from build123d import *

# Parameters (mm, degrees)
SKETCH1_W            = 122
SKETCH1_H            = 101.3
BOSS_EXTRUDE1_DEPTH  = 18
SKETCH2_W            = 118
SKETCH2_H            = 97.3
CUT_EXTRUDE1_DEPTH   = 34
SKETCH4_R            = 5.953519792
CUT_EXTRUDE5_DEPTH   = 2
SKETCH5_W            = 41.658553798
SKETCH5_H            = 19.550778972
CUT_EXTRUDE10_DEPTH  = 2
SKETCH9_W            = 11.907039584
SKETCH9_H            = 11.615
CUT_EXTRUDE12_DEPTH  = 5
SKETCH10_W           = 11.907039584
SKETCH10_H           = 11.615
CUT_EXTRUDE13_DEPTH  = 5
SKETCH11_R           = 1.25
BOSS_EXTRUDE6_DEPTH  = 17
SKETCH14_R           = 1.25
BOSS_EXTRUDE8_DEPTH  = 17
SKETCH15_R           = 1.25
BOSS_EXTRUDE10_DEPTH = 17
SKETCH16_W           = 14.214546847
SKETCH16_H           = 17.568519792
CUT_EXTRUDE14_DEPTH  = 5
SKETCH17_R           = 1.6
BOSS_EXTRUDE11_DEPTH = 1
BOSS_EXTRUDE11_TAPER = 20
SKETCH18_R           = 1.6
BOSS_EXTRUDE13_DEPTH = 1
BOSS_EXTRUDE13_TAPER = 20
SKETCH19_R           = 1.513275
BOSS_EXTRUDE14_DEPTH = 1
BOSS_EXTRUDE14_TAPER = 20


with BuildPart() as part:
    # Sketch1 → Boss-Extrude1 (new, symmetric)
    with BuildSketch(Plane.XY):
        with Locations((129.5, -82.15)):
            Rectangle(SKETCH1_W, SKETCH1_H)
    extrude(amount=BOSS_EXTRUDE1_DEPTH, both=True)

    # Sketch2 → Cut-Extrude1 (cut)
    with BuildSketch(Plane.XY.offset(18)):
        with Locations((129.5, -82.15)):
            Rectangle(SKETCH2_W, SKETCH2_H)
    extrude(amount=-CUT_EXTRUDE1_DEPTH, mode=Mode.SUBTRACT)

    # Sketch4 → Cut-Extrude5 (cut)
    with BuildSketch(Plane(origin=(0, -132.8, 0), x_dir=(-1, 0, 0), z_dir=(0, -1, 0))):
        with Locations(Location((-132.2, -6.385, 0), (0, 0, 90))):
            Circle(SKETCH4_R)
        with Locations(Location((-146.414546847, -6.385, 0), (0, 0, 90))):
            Circle(SKETCH4_R)
    extrude(amount=-CUT_EXTRUDE5_DEPTH, mode=Mode.SUBTRACT)

    # Sketch5 → Cut-Extrude10 (cut)
    with BuildSketch(Plane(origin=(0, -132.8, 0), x_dir=(-1, 0, 0), z_dir=(0, -1, 0))):
        with Locations((-96.070620406, -8.224610514)):
            Rectangle(SKETCH5_W, SKETCH5_H)
    extrude(amount=-CUT_EXTRUDE10_DEPTH, mode=Mode.SUBTRACT)

    # Sketch9 → Cut-Extrude12 (cut)
    with BuildSketch(Plane(origin=(0, -132.8, 0), x_dir=(-1, 0, 0), z_dir=(0, -1, 0))):
        with Locations((-146.414546847, -12.1925)):
            Rectangle(SKETCH9_W, SKETCH9_H)
    extrude(amount=-CUT_EXTRUDE12_DEPTH, mode=Mode.SUBTRACT)

    # Sketch10 → Cut-Extrude13 (cut)
    with BuildSketch(Plane(origin=(0, -132.8, 0), x_dir=(-1, 0, 0), z_dir=(0, -1, 0))):
        with Locations((-132.2, -12.1925)):
            Rectangle(SKETCH10_W, SKETCH10_H)
    extrude(amount=-CUT_EXTRUDE13_DEPTH, mode=Mode.SUBTRACT)

    # Sketch11 → Boss-Extrude6 (add)
    with BuildSketch(Plane.XY.offset(-16)):
        with Locations((91.5, -40.5)):
            Circle(SKETCH11_R)
    extrude(amount=BOSS_EXTRUDE6_DEPTH)

    # Sketch14 → Boss-Extrude8 (add)
    with BuildSketch(Plane.XY.offset(-16)):
        with Locations((166.43, -40.5)):
            Circle(SKETCH14_R)
    extrude(amount=BOSS_EXTRUDE8_DEPTH)

    # Sketch15 → Boss-Extrude10 (add)
    with BuildSketch(Plane.XY.offset(-16)):
        with Locations((180.9, -126.3)):
            Circle(SKETCH15_R)
    extrude(amount=BOSS_EXTRUDE10_DEPTH)

    # Sketch16 → Cut-Extrude14 (cut)
    with BuildSketch(Plane(origin=(0, -132.8, 0), x_dir=(-1, 0, 0), z_dir=(0, -1, 0))):
        with Locations((-139.307273424, -9.215740104)):
            Rectangle(SKETCH16_W, SKETCH16_H)
    extrude(amount=-CUT_EXTRUDE14_DEPTH, mode=Mode.SUBTRACT)

    # Sketch17 → Boss-Extrude11 (add)
    with BuildSketch(Plane.XY.offset(-16)):
        with Locations((91.5, -40.5)):
            Circle(SKETCH17_R)
    extrude(amount=BOSS_EXTRUDE11_DEPTH, taper=BOSS_EXTRUDE11_TAPER)

    # Sketch18 → Boss-Extrude13 (add)
    with BuildSketch(Plane.XY.offset(-16)):
        with Locations((166.43, -40.5)):
            Circle(SKETCH18_R)
    extrude(amount=BOSS_EXTRUDE13_DEPTH, taper=BOSS_EXTRUDE13_TAPER)

    # Sketch19 → Boss-Extrude14 (add)
    with BuildSketch(Plane.XY.offset(-16)):
        with Locations((180.9, -126.3)):
            Circle(SKETCH19_R)
    extrude(amount=BOSS_EXTRUDE14_DEPTH, taper=BOSS_EXTRUDE14_TAPER)


solid = part.part
CAD build for the part. Positions are in the model's coordinates, mm. A direction names the side the tool comes from. Coordinates: 2 decimals unless noted, no trailing zeros. Order: outer loops, then holes, each group sorted by start corner. A loop starts at its lowest first (then second) coordinate and runs counter-clockwise, first axis right, second up. Notation, with made-up numbers: (49.5, -16.75) -> (89.5, -16.75) arc R10 cw to (89.5, -2.75) -> close; hole circle Ø11 at (80.5, -15.5). An arc over 180 degrees is marked (long way). Answer in a Markdown table with one row per item.
1) Band-saw the part on B-B (z = 12). List the corners of the cut face in (x, y), and give its area (3 significant figures).
Check values:
| item | result |
|---|---|
| outline | (68.5, -132.8) -> (75.24, -132.8) -> (75.24, -130.8) -> (70.5, -130.8) -> (70.5, -33.5) -> (188.5, -33.5) -> (188.5, -130.8) -> (152.37, -130.8) -> (152.37, -132.8) -> (190.5, -132.8) -> (190.5, -31.5) -> (68.5, -31.5) -> close; (116.9, -132.8) -> (126.25, -132.8) -> (126.25, -130.8) -> (116.9, -130.8) -> close |
| area | 742 mm2 |
2) Drill centre lines: line 1 (Y direction, x = 183.5, z = -12.5); line 2 (X direction, y = -117, z = 6); line 3 (Y direction, x = 167.5, z = 0). Where is each one in solid material? Low to high.
Check values:
| item | result |
|---|---|
| line 1 | -132.8 to -130.8, -33.5 to -31.5 |
| line 2 | 68.5 to 70.5, 188.5 to 190.5 |
| line 3 | -132.8 to -130.8, -41.15 to -39.85, -33.5 to -31.5 |
3) Band-saw the part on A-A (z = -11). List the corners of the cut face in (x, y).
Check values:
| item | result |
|---|---|
| outline | (68.5, -132.8) -> (190.5, -132.8) -> (190.5, -31.5) -> (68.5, -31.5) -> close; circle Ø2.5 at (91.5, -40.5); circle Ø2.5 at (166.43, -40.5); circle Ø2.5 at (180.9, -126.3); hole (70.5, -130.8) -> (188.5, -130.8) -> (188.5, -33.5) -> (70.5, -33.5) -> close |
4) Flat gauge pins, fed straight in: P1, Ø2, axis at x = 90.5, y = -104.5, coming from the +Z side; P2, Ø1, axis at x = 137, y = -132, coming from the +Z side; P3, Ø1.2, axis at x = 181.5, y = -126, coming from the +Z side. Where does each tip first touch, or does it go through?
Check values:
| item | result |
|---|---|
| P1 | z = -16 |
| P2 | z = 0.43 |
| P3 | z = 1 |
5) Band-saw the part on C-C (x = 157). List the corners of the cut face in (y, z).
Check values:
| item | result |
|---|---|
| outline | (-132.8, -18) -> (-31.5, -18) -> (-31.5, 18) -> (-33.5, 18) -> (-33.5, -16) -> (-130.8, -16) -> (-130.8, 18) -> (-132.8, 18) -> close |
6) Band-saw the part on D-D (y = -102.5). List the corners of the cut face in (x, z).
Check values:
| item | result |
|---|---|
| outline | (68.5, -18) -> (190.5, -18) -> (190.5, 18) -> (188.5, 18) -> (188.5, -16) -> (70.5, -16) -> (70.5, 18) -> (68.5, 18) -> close |
7) Which spindle directions (+Z, -Z, +X, -X, +Y, -Y) get a long thin tool onto all of the face, cutting with end or side? Do faces 4 (the face through (179.979, -125.455, -7.252)), 5 (the face through (127.944, -131.814, 2.222)), 6 (the face through (129, -31.5, 0)). Say none if no direction does.
Check values:
| item | result |
|---|---|
| face 4 | +Z |
| face 5 | +Z, -Y |
| face 6 | +Z, -Z, +X, -X, +Y |
8) Mould opens along X. For faces 1 (the face through (150.58, -131.81, 2.13)), 2 (the face through (129, -81, -18)), 3 (the face through (68.5, -83, 0)) say: pulls with the +X half, pulls with the -X half, needs draft (parallel to the pull), parting line crosses it, or undercut.
Check values:
| item | result |
|---|---|
| face 1 | undercut |
| face 2 | needs draft |
| face 3 | pulls with the -X half |
